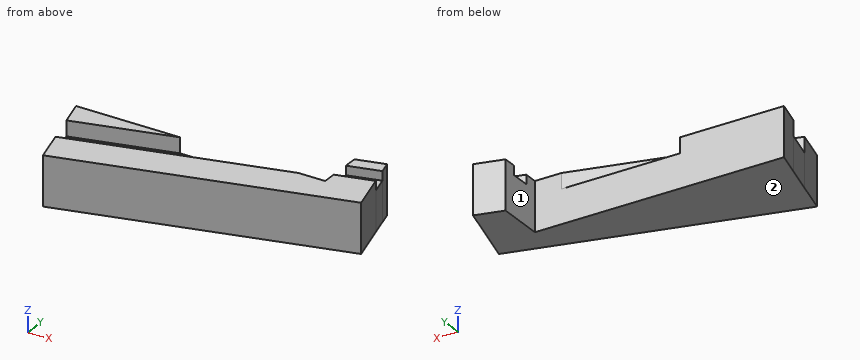
```python
from build123d import *

# Parameters (mm, degrees)
F4_DEPTH = 16
F5_DEPTH = 11
F6_DEPTH = 13


with BuildPart() as f4:
    # F2 (on Top) → F4 (new body)
    with BuildSketch(Plane.XY):
        Polygon((11.7414596618, 0.0402860931), (0, -3.1058285412), (0, -7.5), (-8.671864531, -7.5), (-76.4647760054, -25.6650558821), (-73.5208917648, -36.6517814396), (15.2029819926, -12.8782911169), align=None)
    extrude(amount=F4_DEPTH)



with BuildPart() as f4b:
    # F2 (on Top) → F4, piece 2 (new body)
    with BuildSketch(Plane.XY):
        Polygon((-79.0529664564, -16.0057976192), (-47.3088975825, -7.5), (-81.3320880594, -7.5), align=None)
    extrude(amount=F4_DEPTH)


with BuildPart() as f4c:
    # F2 (on Top) → F4, piece 3 (new body)
    with BuildSketch(Plane.XY):
        Polygon((0, 7.5), (0, 3.1058285412), (10.1885453912, 5.8358410508), (9.0900025265, 9.9356588362), align=None)
    extrude(amount=F4_DEPTH)


with BuildPart() as f4_1:
    add(f4.part)

    add(f4b.part)  # F5 merges F4b
    # F2 (on Top) → F5 (join)
    with BuildSketch(Plane.XY):
        Polygon((-76.4647760054, -25.6650558821), (-8.671864531, -7.5), (-47.3088975825, -7.5), (-79.0529664564, -16.0057976192), align=None)
    extrude(amount=F5_DEPTH)


    add(f4c.part)  # F6 merges F4c
    # F2 (on Top) → F6 (join)
    with BuildSketch(Plane.XY):
        Polygon((0, 3.1058285412), (0, 0), (0, -3.1058285412), (11.7414596618, 0.0402860931), (10.1885453912, 5.8358410508), align=None)
    extrude(amount=F6_DEPTH)


solid = f4_1.part
```
Geometry: final body of the model. Coordinates: model frame, mm. Face numbers are marked on the shaded views. A direction names the side the tool comes from. Round coordinates to 2 decimals unless told otherwise and drop trailing zeros. Write each loop counter-clockwise with the first axis right and the second up, starting at its lowest first coordinate (ties: lowest second). Pieces come first, ordered by that corner, then holes.
Item 1: Set-up query: the marked faces 1 and 2. Return all of +Z, -Z, +X, -X, +Y, -Y with unobstructed straight access to the full face (end or side cutting, diameter ignored); none if empty.
Item 2: Section query B-B (z = 4.75). Return loops of the section in (x, y).
Item 3: Section query C-C (y = -12). Return loops of the section in (x, z), plus the area to 3 significant figures.
Item 4: Section query D-D (x = -66). Return loops of the section in (y, z).
Item 5: Material intervals for L1, parallel to Z at x = -47, y = -10; L2, parallel to Y at x = -57, z = 12.5; L3, parallel to Y at x = -20.5, z = 7, sorted ascending.
Item 6: Section query A-A (z = 14.75). Return loops of the section in (x, y).
Item 7: Pin query (flat end, axial travel): P1, Ø2, axis at x = -35.5, y = -7.5, coming from the +Z side; P2, Ø5, axis at x = 1, z = 12, coming from the -Y side; P3, Ø6, axis at y = -24.5, z = 9.5, coming from the -X side. Return the tip coordinate at first contact, or that it passes through.
Completed:
1. face 1: +Z, -Z, -X, +Y
1. face 2: -Z, +X, -X, +Y, -Y
2. outline: (-81.33, -7.5) - (-73.52, -36.65) - (15.2, -12.88) - (9.09, 9.94) - (0, 7.5) - (0, -7.5) - close
3. outline: (-80.13, 0) - (14.97, 0) - (14.97, 16) - (-25.47, 16) - (-25.47, 11) - (-64.1, 11) - (-64.1, 16) - (-80.13, 16) - close
3. area: 1,330 mm2
4. outline: (-34.64, 0) - (-7.5, 0) - (-7.5, 16) - (-12.51, 16) - (-12.51, 11) - (-22.86, 11) - (-22.86, 16) - (-34.64, 16) - close
5. L1: z = 0 to 11
5. L2: y = -32.23 to -20.45, -10.1 to -7.5
5. L3: y = -22.44 to -7.5
6. outline: (-81.33, -7.5) - (-79.05, -16.01) - (-47.31, -7.5) - close; (-76.46, -25.67) - (-73.52, -36.65) - (15.2, -12.88) - (11.74, 0.04) - (0, -3.11) - (0, -7.5) - (-8.67, -7.5) - close; (0, 3.11) - (10.19, 5.84) - (9.09, 9.94) - (0, 7.5) - close
7. P1: stops at z = 11
7. P2: stops at y = -17.35
7. P3: stops at x = -77.58
